Check sheet for the drawn part. Datum: minimum x, y, z corner. Units: mm. A direction names the side the tool comes from. Coordinates: 2 decimals unless noted, no trailing zeros. Order: outer loops, then holes, each group sorted by start corner. A loop starts at its lowest first (then second) coordinate and runs counter-clockwise, first axis right, second up. Notation, with made-up numbers: (-30, 85.25) - (-12, 85.25) arc R22 cw to (-12, 108.25) - close; hole circle Ø11 at (-27.75, 14.25). An arc over 180 degrees is marked (long way). One line per item, written item: value. Start each with the question number.
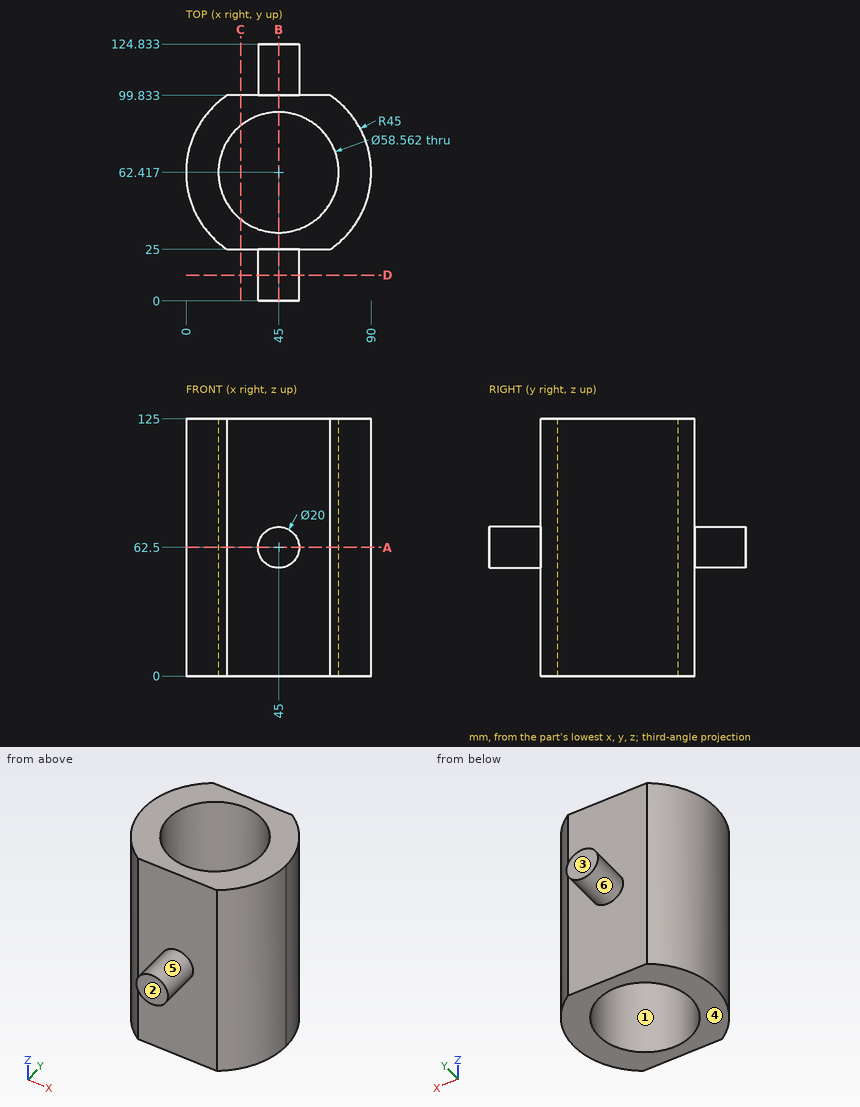
Q1. Cross-section at B-B, the plane x = 45. Enter the section's corners in (y, z) (1 decimal).
Q2. Cross-section at A-A, the plane z = 62.5. Enter the section's corners in (x, y), and give its area (3 significant figures).
Q3. Cross-section at C-C, the plane x = 26.5. Enter the section's corners in (y, z).
Q4. Material ranges on probe 1 along Y at (x, z) = (45, 73) (1 decimal); probe 2 along Y at (x, z) = (45, 57) (1 decimal); probe 3 along X at (y, z) = (53, 57) (1 decimal), recorded low to high.
Q5. Cross-section at D-D, the plane y = 12.5. Enter the section's corners in (x, z).
Q6. Set-up check for the marked faces 4, 5 and 6: record each of +Z, -Z, +X, -X, +Y, -Y from which the full face is reachable in a straight line by a thin tool's end or side.
Q7. Gauge pin test, flat ends, axial feed: P1, Ø2, axis at x = 44, z = 51.5, coming from the -Y side; P2, Ø10, axis at x = 65, y = 72, coming from the +Z side; P3, Ø3, axis at x = 30.5, z = 67, coming from the +Y side; P4, Ø12, axis at y = 108, z = 60, coming from the +X side. Record the tip position at first contact, or that the pin passes through.
Q8. Release check for a two-part mould opening along Y. For the marked faces 1, 2 and 3 record: released by +Y, released by -Y, zero draft, split by the parting line, or undercut.
Check result:
1. outline: (0, 52.5) - (25, 52.5) - (25, 0) - (33.1, 0) - (33.1, 125) - (25, 125) - (25, 72.5) - (0, 72.5) - close; (91.7, 0) - (99.8, 0) - (99.8, 52.5) - (124.8, 52.5) - (124.8, 72.5) - (99.8, 72.5) - (99.8, 125) - (91.7, 125) - close
2. outline: (20, 25) - (35, 25) - (35, 0) - (55, 0) - (55, 25) - (70, 25) arc R45 ccw to (70, 99.83) - (55, 99.83) - (55, 124.83) - (35, 124.83) - (35, 99.83) - (20, 99.83) arc R45 ccw to start; hole circle Ø58.56 at (45, 62.42)
2. area: 4,150 mm2
3. outline: (25, 0) - (39.72, 0) - (39.72, 125) - (25, 125) - close; (85.11, 0) - (99.83, 0) - (99.83, 125) - (85.11, 125) - close
4. probe 1: y = 25 to 33.1, 91.7 to 99.8
4. probe 2: y = 0 to 33.1, 91.7 to 124.8
4. probe 3: x = 1 to 17.3, 72.7 to 89
5. outline: circle Ø20 at (45, 62.5)
6. face 4: -Z, +X, -X, +Y, -Y
6. face 5: -Y
6. face 6: +Y
7. P1: stops at y = 25
7. P2: passes through
7. P3: stops at y = 99.83
7. P4: stops at x = 55
8. face 1: undercut
8. face 2: released by -Y
8. face 3: released by +Y
